CAD build for the part. Positions are in the model's coordinates, mm. Face numbers are marked on the shaded views. A direction names the side the tool comes from. Coordinates: 2 decimals unless noted, no trailing zeros. Order: outer loops, then holes, each group sorted by start corner. A loop starts at its lowest first (then second) coordinate and runs counter-clockwise, first axis right, second up. Notation, with made-up numbers: (-33.5, 84) -> (-8.5, 84) arc R7 cw to (-8.5, 97) -> close; hole circle Ø1 at (-15.75, 74.25). An arc over 180 degrees is marked (long way). Use one line per item in the form item = value. Start each with the question number.
from build123d import *

# Parameters (mm, degrees)
SALIENTE_EXTRUIR2_DEPTH = 20
CROQUIS5_R              = 2
CORTAR_EXTRUIR2_DEPTH   = 98.867257037


with BuildPart() as part:
    # Croquis1 → Saliente-Extruir2 (new body)
    with BuildSketch(Plane.XY):
        with BuildLine():
            Line((-57, 0), (-55.991070717, 0))
            ThreePointArc((-55.991070717, 0), (-55.290305828, -0.286607702), (-54.991230168, -0.982142857))
            ThreePointArc((-54.991230168, -0.982142857), (0, -55), (54.991230168, -0.982142857))
            ThreePointArc((54.991230168, -0.982142857), (55.290305828, -0.286607702), (55.991070717, 0))
            Line((55.991070717, 0), (57, 0))
            Line((57, 0), (76.5, 0))
            ThreePointArc((76.5, 0), (76.853553391, -0.146446609), (77, -0.5))
            Line((77, -0.5), (77, -1.5))
            ThreePointArc((77, -1.5), (76.853553391, -1.853553391), (76.5, -2))
            Line((76.5, -2), (57.92236183, -2))
            ThreePointArc((57.92236183, -2), (57.233785087, -2.274836523), (56.923700419, -2.948275862))
            ThreePointArc((56.923700419, -2.948275862), (0, -57), (-56.923700419, -2.948275862))
            ThreePointArc((-56.923700419, -2.948275862), (-57.233785087, -2.274836523), (-57.92236183, -2))
            Line((-57.92236183, -2), (-76.5, -2))
            ThreePointArc((-76.5, -2), (-76.853553391, -1.853553391), (-77, -1.5))
            Line((-77, -1.5), (-77, -0.5))
            ThreePointArc((-77, -0.5), (-76.853553391, -0.146446609), (-76.5, 0))
            Line((-76.5, 0), (-57, 0))
        make_face()
    extrude(amount=SALIENTE_EXTRUIR2_DEPTH)

    # Croquis5 → Cortar-Extruir2 (cut, symmetric)
    with BuildSketch(Plane(origin=(0, 0, 0), x_dir=(1, 0, 0), z_dir=(0, 1, 0))):
        with Locations(Location((67, -10, 0), (0, 0, 270))):
            Circle(CROQUIS5_R)
    cortar_extruir2 = extrude(amount=CORTAR_EXTRUIR2_DEPTH, both=True, mode=Mode.SUBTRACT)

    # Simetría4: Cortar-Extruir2 across plane
    add(cortar_extruir2.mirror(Plane(origin=(0, 0, 0), x_dir=(0, 0, 1), z_dir=(1, 0, 0))), mode=Mode.SUBTRACT)


solid = part.part
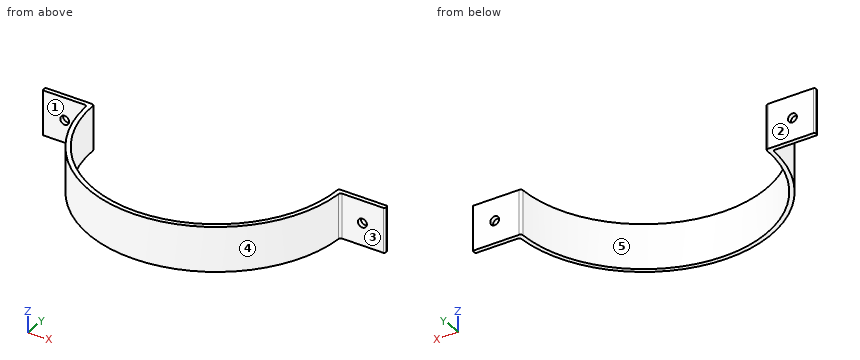
1) Cut at B-B on x = 67. Give the cut face in (y, z), then the cut area to 3 significant figures.
2) Probe L1, parallel to X at y = -0.8, z = 10; L2, parallel to X at y = -0.45, z = 10; L3, parallel to Y at x = -62.5, z = 7.25. List the from-to ranges inside material, lowest first.
3) Cut at D-D on z = 18.25. Give the cut face in (x, y).
4) Cut at A-A on z = 10. Give the cut face in (x, y), then the cut area to 3 significant figures.
5) Two-plate mould, pull along X, no slides. Class the marked faces 3, 4 and 5: released by +X, released by -X, zero draft, split by the parting line, or undercut.
6) 3-axis set-ups, long thin cutter, end or side, ignore diameter. For the marked faces 1 and 2: which of +Z, -Z, +X, -X, +Y, -Y reach the whole face in a straight line?
7) Cut at C-C on y = -8.5. Give the cut face in (x, z).
8) Drop flat-ended pins along their axis: P1, Ø4.5, axis at x = 67, z = 10, coming from the -Y side; P2, Ø4.5, axis at x = -67, z = 10, coming from the +Y side; P3, Ø3, axis at y = -12, z = 14.5, coming from the -X side; P4, Ø4, axis at y = -18, z = 14, coming from the -X side. Give the stop position or say it passes through.
Values follow:
q1.outline = (-2, 0) -> (0, 0) -> (0, 8) -> (-2, 8) -> close; (-2, 12) -> (0, 12) -> (0, 20) -> (-2, 20) -> close
q1.area = 32.0 mm^2
q2.L1 = -77 to -69, -65 to -55.01, 55.01 to 65, 69 to 77
q2.L2 = -77 to -69, -65 to -55.16, 55.16 to 65, 69 to 77
q2.L3 = -2 to 0
q3.outline = (-77, -1.5) arc R0.5 ccw to (-76.5, -2) -> (-57.92, -2) arc R1 cw to (-56.92, -2.95) arc R57 ccw to (56.92, -2.95) arc R1 cw to (57.92, -2) -> (76.5, -2) arc R0.5 ccw to (77, -1.5) -> (77, -0.5) arc R0.5 ccw to (76.5, 0) -> (55.99, 0) arc R1 ccw to (54.99, -0.98) arc R55 cw to (-54.99, -0.98) arc R1 ccw to (-55.99, 0) -> (-76.5, 0) arc R0.5 ccw to (-77, -0.5) -> close
q4.outline = (-77, -1.5) arc R0.5 ccw to (-76.5, -2) -> (-69, -2) -> (-69, 0) -> (-76.5, 0) arc R0.5 ccw to (-77, -0.5) -> close; (-65, -2) -> (-57.92, -2) arc R1 cw to (-56.92, -2.95) arc R57 ccw to (56.92, -2.95) arc R1 cw to (57.92, -2) -> (65, -2) -> (65, 0) -> (55.99, 0) arc R1 ccw to (54.99, -0.98) arc R55 cw to (-54.99, -0.98) arc R1 ccw to (-55.99, 0) -> (-65, 0) -> close; (69, -2) -> (76.5, -2) arc R0.5 ccw to (77, -1.5) -> (77, -0.5) arc R0.5 ccw to (76.5, 0) -> (69, 0) -> close
q4.area = 416 mm^2
q5.face_3 = zero draft
q5.face_4 = split by the parting line
q5.face_5 = undercut
q6.face_1 = +Z, -Z, -X, -Y
q6.face_2 = +Z, -Z, +X, -X, +Y
q7.outline = (-56.36, 0) -> (-54.34, 0) -> (-54.34, 20) -> (-56.36, 20) -> close; (54.34, 0) -> (56.36, 0) -> (56.36, 20) -> (54.34, 20) -> close
q8.P1 = -2
q8.P2 = 0
q8.P3 = -56.02
q8.P4 = -54.71
